```python
from build123d import *

# Parameters (mm, degrees)
SKETCH2_R               = 20
BOSS_EXTRUDE1_DEPTH     = 2
CUT_EXTRUDE2_DEPTH      = 46.628938186
CUT_EXTRUDE2_DEPTH_BACK = 46.628938186
SKETCH6_R               = 25.059608459
SKETCH6_R_2             = 6.28
SKETCH3_R               = 7.4
SKETCH3_R_2             = 5.9
BOSS_EXTRUDE2_DEPTH     = 1
SKETCH7_R               = 13.022061682
CUT_EXTRUDE3_DEPTH      = 1


with BuildPart() as part:
    # Sketch2 → Boss-Extrude1 (new body)
    with BuildSketch(Plane(origin=(0, 0, 0), x_dir=(1, 0, 0), z_dir=(0, 0.7071067811865464, 0.7071067811865488))):
        with Locations(Location((0, 20, 0), (0, 0, 270))):
            Circle(SKETCH2_R)
    extrude(amount=-BOSS_EXTRUDE1_DEPTH)

    # Sketch6 → Cut-Extrude2 (cut, two sides: drawn at the far end of the back side and taken through both)
    with BuildSketch(Plane(origin=(0, 0, 0), x_dir=(1, 0, 0), z_dir=(0, 1, 0)).offset(-CUT_EXTRUDE2_DEPTH_BACK)):
        with Locations((0, 9)):
            Circle(SKETCH6_R)
        with Locations(Location((0, 9, 0), (0, 0, 90))):
            Circle(SKETCH6_R_2, mode=Mode.SUBTRACT)
    extrude(amount=CUT_EXTRUDE2_DEPTH + CUT_EXTRUDE2_DEPTH_BACK, mode=Mode.SUBTRACT)


with BuildPart() as body_2:
    # Sketch3 → Boss-Extrude2 (new body)
    with BuildSketch(Plane(origin=(0, -3.25, 0), x_dir=(1, 0, 0), z_dir=(0, 1, 0))):
        with Locations(Location((0, 7.4, 0), (0, 0, 270))):
            Circle(SKETCH3_R)
        with Locations(Location((0, 7.4, 0), (0, 0, 270))):
            Circle(SKETCH3_R_2, mode=Mode.SUBTRACT)
    extrude(amount=BOSS_EXTRUDE2_DEPTH)

    # Sketch7 → Cut-Extrude3 (cut)
    with BuildSketch(Plane.XZ.offset(3.25)):
        with Locations((0.290894274, -7.517427113)):
            Circle(SKETCH7_R)
    extrude(amount=-CUT_EXTRUDE3_DEPTH, mode=Mode.SUBTRACT)


solid = part.part
```
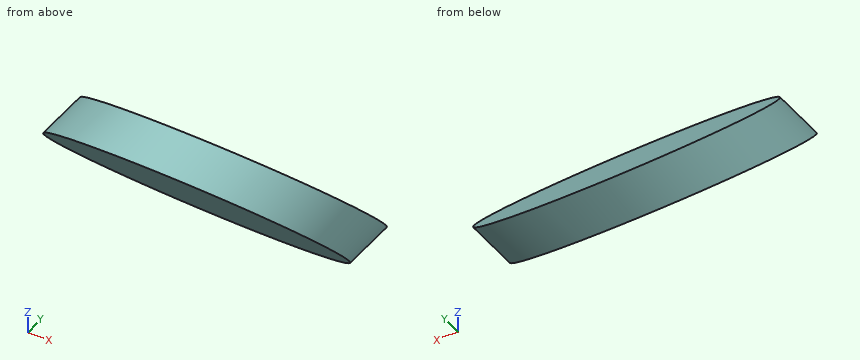
Part model, mm, in its own coordinate system. Round coordinates to 2 decimals unless told otherwise and drop trailing zeros. Write each loop counter-clockwise with the first axis right and the second up, starting at its lowest first coordinate (ties: lowest second). Pieces come first, ordered by that corner, then holes. Notation, with made-up numbers: (30.25, 20) -> (61.25, 20) arc R31 cw to (61.25, 57) -> close; hole circle Ø6 at (3, 70.5). An arc over 180 degrees is marked (long way). Return JSON: item names as keys, results as strings. Group by question number.
Q1. Saw through at C-C on y = 13.75. Write the cut outline in (x, z), plus the area to 3 significant figures.
Q2. Saw through at B-B on z = -9. Write the cut outline in (x, y), plus the area to 3 significant figures.
Q3. Probe L1, parallel to Y at x = -2.5, z = -8.5; L2, parallel to Y at x = 3.5, z = -6.75; L3, parallel to Z at x = -4.25, y = 7.25. List the from-to ranges inside material, lowest first. Write a range as [from, to].
Q4. Saw through at A-A on x = 0. Write the cut outline in (y, z).
Q5. Pin check, flat tips, straight feed: pin 1 (1.5 mm diameter, centred on x = 2.5, z = -7.5, fed in from -Y); pin 2 (1 mm diameter, centred on x = 4, z = -11, fed in from +Y); pin 3 (1 mm diameter, centred on x = -0.5, z = -8.5, fed in from +Y). Stop position of each tip, or through.
Answer:
{
 "1": {"outline": "(-4.11, -13.75) arc R6.28 ccw to (4.11, -13.75) -> close", "area": "8.61 mm2"},
 "2": {"outline": "(-6.28, 6.17) -> (6.28, 6.17) -> (6.28, 9) -> (-6.28, 9) -> close", "area": "35.5 mm2"},
 "3": {"L1": "[5.67, 8.5]", "L2": "[3.92, 6.75]", "L3": "[-10.08, -7.25]"},
 "4": {"outline": "(-0.11, -2.72) -> (12.45, -15.28) -> (15.28, -15.28) -> (2.72, -2.72) -> close"},
 "5": {"pin 1": "y = 3.92", "pin 2": "y = 11.5", "pin 3": "y = 9"}
}
